```python
from build123d import *

# Parameters (mm, degrees)
BOSS_EXTRUDE1_DEPTH      = 23
BOSS_EXTRUDE1_DEPTH_BACK = 23
CUT_EXTRUDE1_REACH       = 32.068
SKETCH6_R                = 2.5


with BuildPart() as part:
    # Sketch1 → Boss-Extrude1 (new, two sides: drawn at the far end of the back side and taken through both)
    with BuildSketch(Plane.XY.offset(-BOSS_EXTRUDE1_DEPTH_BACK)):
        Polygon((-15, 6.25), (-15, 3.25), (-6, 3.25), (-6, -6), (6, -6), (6, 3.25), (15, 3.25), (15, 6.25), align=None)
    extrude(amount=BOSS_EXTRUDE1_DEPTH + BOSS_EXTRUDE1_DEPTH_BACK)

    # Sketch2 → Revolve1 (revolve)
    with BuildSketch(Plane.XY.offset(19), mode=Mode.PRIVATE) as revolve1_sk:
        Polygon((10.5, -3.125), (10.5, -5.375), (9.5, -5.375), (9.5, -4.625), (7, -4.625), (7, -5.625), (6, -5.625), (6, -4.625), (-6, -4.625), (-6, -5.625), (-7, -5.625), (-7, -4.625), (-9.5, -4.625), (-9.5, -5.375), (-10.5, -5.375), (-10.5, -3.125), align=None)
    revolve(revolve1_sk.sketch.rotate(Axis((-10.5, -3.125, 19), (1, 0, 0)), 90), axis=Axis((-10.5, -3.125, 19), (1, 0, 0)))

    # Sketch3 → Revolve2 (revolve)
    with BuildSketch(Plane.XY.offset(-19), mode=Mode.PRIVATE) as revolve2_sk:
        Polygon((10.5, -3.125), (10.5, -5.375), (9.5, -5.375), (9.5, -4.625), (7, -4.625), (7, -5.625), (6, -5.625), (6, -4.625), (-6, -4.625), (-6, -5.625), (-7, -5.625), (-7, -4.625), (-9.5, -4.625), (-9.5, -5.375), (-10.5, -5.375), (-10.5, -3.125), align=None)
    revolve(revolve2_sk.sketch.rotate(Axis((-10.5, -3.125, -19), (1, 0, 0)), 90), axis=Axis((-10.5, -3.125, -19), (1, 0, 0)))

    # Sketch4 → Cut-Revolve1 (revolve, cut)
    with BuildSketch(Plane(origin=(0, 0, 0), x_dir=(0, 0, -1), z_dir=(1, 0, 0)), mode=Mode.PRIVATE) as cut_revolve1_sk:
        Polygon((-14, 6.25), (-11.5, 6.25), (-11.933, 5.817), (-11.933, -5.567), (-11.5, -6), (-14, -6), align=None)
    revolve(cut_revolve1_sk.sketch.rotate(Axis((0, -6, 14), (0, 1, 0)), 180), axis=Axis((0, -6, 14), (0, 1, 0)), mode=Mode.SUBTRACT)

    # Sketch5 → Cut-Revolve2 (revolve, cut)
    with BuildSketch(Plane(origin=(0, 0, 0), x_dir=(0, 0, -1), z_dir=(1, 0, 0)), mode=Mode.PRIVATE) as cut_revolve2_sk:
        Polygon((14, 6.25), (16.5, 6.25), (16.067, 5.817), (16.067, -5.567), (16.5, -6), (14, -6), align=None)
    revolve(cut_revolve2_sk.sketch.rotate(Axis((0, -6, -14), (0, 1, 0)), 180), axis=Axis((0, -6, -14), (0, 1, 0)), mode=Mode.SUBTRACT)

    # Sketch6 → Cut-Extrude1 (cut, up to next)
    with BuildSketch(Plane(origin=(0, 6.25, 0), x_dir=(1, 0, 0), z_dir=(0, 1, 0)), mode=Mode.PRIVATE) as cut_extrude1_sk1:
        with Locations(Location((-10, 16, 0), (0, 0, 270))):
            Circle(SKETCH6_R)
    cut_extrude1_tool1 = extrude(cut_extrude1_sk1.sketch, amount=-CUT_EXTRUDE1_REACH, mode=Mode.PRIVATE) & part.part
    # Sketch6 → Cut-Extrude1 (cut, up to next)
    with BuildSketch(Plane(origin=(0, 6.25, 0), x_dir=(1, 0, 0), z_dir=(0, 1, 0)), mode=Mode.PRIVATE) as cut_extrude1_sk2:
        with Locations(Location((10, 16, 0), (0, 0, 270))):
            Circle(SKETCH6_R)
    cut_extrude1_tool2 = extrude(cut_extrude1_sk2.sketch, amount=-CUT_EXTRUDE1_REACH, mode=Mode.PRIVATE) & part.part
    # Sketch6 → Cut-Extrude1 (cut, up to next)
    with BuildSketch(Plane(origin=(0, 6.25, 0), x_dir=(1, 0, 0), z_dir=(0, 1, 0)), mode=Mode.PRIVATE) as cut_extrude1_sk3:
        with Locations(Location((-10, -16, 0), (0, 0, 270))):
            Circle(SKETCH6_R)
    cut_extrude1_tool3 = extrude(cut_extrude1_sk3.sketch, amount=-CUT_EXTRUDE1_REACH, mode=Mode.PRIVATE) & part.part
    # Sketch6 → Cut-Extrude1 (cut, up to next)
    with BuildSketch(Plane(origin=(0, 6.25, 0), x_dir=(1, 0, 0), z_dir=(0, 1, 0)), mode=Mode.PRIVATE) as cut_extrude1_sk4:
        with Locations(Location((10, -16, 0), (0, 0, 270))):
            Circle(SKETCH6_R)
    cut_extrude1_tool4 = extrude(cut_extrude1_sk4.sketch, amount=-CUT_EXTRUDE1_REACH, mode=Mode.PRIVATE) & part.part
    add(cut_extrude1_tool1.solids().sort_by_distance((-10, 6.25, -16))[0], mode=Mode.SUBTRACT)
    add(cut_extrude1_tool2.solids().sort_by_distance((10, 6.25, -16))[0], mode=Mode.SUBTRACT)
    add(cut_extrude1_tool3.solids().sort_by_distance((-10, 6.25, 16))[0], mode=Mode.SUBTRACT)
    add(cut_extrude1_tool4.solids().sort_by_distance((10, 6.25, 16))[0], mode=Mode.SUBTRACT)


solid = part.part
```
Design review of the part built by this model. Coordinates are the model's own, in mm. A direction names the side the tool comes from. Give positions to 0.01 mm unless a question says otherwise; leave off trailing zeros. Order: outer loops, then holes, each group sorted by start corner. A loop starts at its lowest first (then second) coordinate and runs counter-clockwise, first axis right, second up. Notation, with made-up numbers: (46.5, -17) -> (62.5, -17) arc R14 ccw to (62.5, 8) -> close; hole circle Ø4 at (39, 47.25). An arc over 180 degrees is marked (long way). Write item = value, one per line. Start each with the question number.
(1) For pin 1 (1.5 mm diameter, centred on y = -3, z = -19, fed in from -X); pin 2 (2 mm diameter, centred on x = -10, y = -4, fed in from -Z); pin 3 (5 mm diameter, centred on y = -2, z = 18.5, fed in from +X), all flat-tipped, find the tip position at first contact; note any pin that passes through.
(2) We need section D-D on z = -14. Write out the cut boundary in (x, y).
(3) We need section B-B on y = 4.5. Write out the cut boundary in (x, z), plus the area to 3 significant figures.
(4) We need section A-A on x = 0. Write out the cut boundary in (y, z), plus the area to 3 significant figures.
(5) Mouldability with a two-part tool opening along X and no side actions: class faces 4 (the face through (0, -6, 0)), 5 (the face through (-9.5, -5, -19)), 6 (the face through (-10.5, -3, -19)) as +X half, -X half, draft (parallel to the pull), parting line (faces both ways), or undercut.
(6) For faces 1 (the face through (-6, -1, 0)), 2 (the face through (-7, -5, 19)), 3 (the face through (10.5, -3, -19)), list the 3-axis set-ups (+Z, -Z, +X, -X, +Y, -Y) from which the entire face can be reached by the end or side of a thin tool; tool diameter is ignored.
(7) To check wall thickness, follow line 1 along Y through (x, z) = (-12.25, 12.5); line 2 along Z through (x, y) = (-9, 4); line 3 along Z through (x, y) = (-6.75, -1.25). State the ranges of each line that lie inside material, in increasing order.
Numbers:
q1.pin_1 = -10.5
q1.pin_2 = -21.25
q1.pin_3 = 10.5
q2.outline = (-15, 3.25) -> (-11.5, 3.25) -> (-11.5, 6.25) -> (-15, 6.25) -> close; (-8.5, 3.25) -> (-6, 3.25) -> (-6, -6) -> (-2.5, -6) -> (-2.07, -5.57) -> (-2.07, 5.82) -> (-2.5, 6.25) -> (-8.5, 6.25) -> close; (2.07, -5.57) -> (2.5, -6) -> (6, -6) -> (6, 3.25) -> (8.5, 3.25) -> (8.5, 6.25) -> (2.5, 6.25) -> (2.07, 5.82) -> close; (11.5, 3.25) -> (15, 3.25) -> (15, 6.25) -> (11.5, 6.25) -> close
q3.outline = (-15, -23) -> (15, -23) -> (15, 23) -> (-15, 23) -> close; hole circle Ø5 at (-10, -16); hole circle Ø5 at (-10, 16); hole circle Ø4.13 at (0, -14); hole circle Ø4.13 at (0, 14); hole circle Ø5 at (10, -16); hole circle Ø5 at (10, 16)
q3.area = 1,270 mm^2
q4.outline = (-6, -23) -> (6.25, -23) -> (6.25, -16.5) -> (5.82, -16.07) -> (-5.57, -16.07) -> (-6, -16.5) -> close; (-6, -11.5) -> (-5.57, -11.93) -> (5.82, -11.93) -> (6.25, -11.5) -> (6.25, 11.5) -> (5.82, 11.93) -> (-5.57, 11.93) -> (-6, 11.5) -> close; (-6, 16.5) -> (-5.57, 16.07) -> (5.82, 16.07) -> (6.25, 16.5) -> (6.25, 23) -> (-6, 23) -> close
q4.area = 461 mm^2
q5.face_4 = draft
q5.face_5 = undercut
q5.face_6 = -X half
q6.face_1 = -X
q6.face_2 = none
q6.face_3 = +Z, -Z, +X, -Y
q7.line_1 = 3.25 to 6.25
q7.line_2 = -23 to -18.29, -13.71 to 13.71, 18.29 to 23
q7.line_3 = -20.65 to -17.35, 17.35 to 20.65
